Autodesk Fusion 360 part; units mm, degrees
sketch "Esquisse1" plane through (0, 0, 0) normal (0, 0, 1) x (1, 0, 0)
  line L0 (0, 0) -> (200, 0)
  line L1 (200, 0) -> (200, 200)
  line L2 (200, 200) -> (0, 200)
  line L3 (0, 200) -> (0, 0)
  dimension "d18" = 200
  dimension "d19" = 200
extrude "Extrusion1" add sketch "Esquisse1" along normal blind 4
chamfer "Chanfrein1" distance 4 angle 45 1 faces at (66.6667, 133.3333, 0)
sketch "Esquisse2" plane through (0, 0, 4) normal (0, 0, 1) x (-1, 0, 0)
  circle A0 centre (-20, -180) radius 2
  circle A1 centre (-180, -180) radius 2
  circle A2 centre (-180, -20) radius 2
  circle A3 centre (-20, -20) radius 2
  line L0 (0, 0) -> (-20, -20)
  line L1 (-200, 0) -> (-180, -20)
  line L2 (0, -200) -> (-20, -180)
  line L3 (-200, -200) -> (-180, -180)
  line L4 (0, -200) -> (0, 0)
  line L5 (0, 0) -> (-200, 0)
  line L6 (-200, 0) -> (-200, -200)
  line L7 (-200, -200) -> (0, -200)
  dimension "d10" = 4
  dimension "d11" = 4
  dimension "d12" = 4
  dimension "d13" = 4
  dimension "d20" = 28.2843
  dimension "d23" = 28.2843
  dimension "d24" = 28.2843
  dimension "d25" = 28.2843
extrude "Extrusion2" cut sketch "Esquisse2" against normal blind 14 contours A0 | A3 | A2 | A1
thread "Filetage1" thread offset 0 thread length 10
thread "Filetage2" thread offset 0 thread length 10
thread "Filetage3" thread offset 0 thread length 10
thread "Filetage4" thread offset 0 thread length 10
equation "d20 = ( sqrt(800) ) * 1 mm"
equation "d23 = ( sqrt(800) ) * 1 mm"
equation "d24 = ( sqrt(800) ) * 1 mm"
equation "d25 = ( sqrt(800) ) * 1 mm"
CAD build for the part. Positions are in the model's coordinates, mm. Coordinates: 2 decimals unless noted, no trailing zeros. Loops run counter-clockwise (first coordinate to the right, second up) from the corner with the lowest first, then second, coordinate; pieces in that order, holes last. Notation, with made-up numbers: (62, 32.25) - (110, 32.25) arc R27 ccw to (110, 63.25) - close; hole circle Ø2 at (24, -13). An arc over 180 degrees is marked (long way). Return JSON: item names as keys, results as strings.
1. Drop flat-ended pins along their axis: pin 1 (1.5 mm diameter, centred on x = 80, z = 1.5, fed in from +Y); pin 2 (2.5 mm diameter, centred on x = 20, y = 180, fed in from +Z). Give the stop position or say it passes through.
Result:
{"pin 1": "stops at y = 198.25", "pin 2": "passes through"}
2. Band-saw the part on A-A (z = 0.8). Give the cut face in (x, y), and give its area (3 significant figures).
Result:
{"outline": "(3.2, 3.2) - (196.8, 3.2) - (196.8, 196.8) - (3.2, 196.8) - close; hole circle Ø4 at (20, 20); hole circle Ø4 at (20, 180); hole circle Ø4 at (180, 20); hole circle Ø4 at (180, 180)", "area": "37,400 mm2"}
3. Probe L1, parallel to X at y = 20, z = 2.25; L2, parallel to Y at x = 180, z = 1.7; L3, parallel to Y at x = 180, z = 1.3. List the from-to ranges inside material, lowest first. Write a range as from..to.
Result:
{"L1": "x = 1.75..18, 22..178, 182..198.25", "L2": "y = 2.3..18, 22..178, 182..197.7", "L3": "y = 2.7..18, 22..178, 182..197.3"}
